```python
from build123d import *

# Parameters (mm, degrees)
SKETCH1_R                                       = 60.5
BOSS_EXTRUDE1_DEPTH                             = 5
SKETCH2_R                                       = 50
SKETCH2_R_2                                     = 45
BOSS_EXTRUDE2_DEPTH                             = 50
SKETCH3_W                                       = 9
SKETCH3_H                                       = 9
BOSS_EXTRUDE3_DEPTH                             = 1
SKETCH3_3_W                                     = 8
SKETCH3_3_H                                     = 9
BOSS_EXTRUDE4_DEPTH                             = 25
SKETCH4_W                                       = 25
SKETCH4_H                                       = 9
BOSS_EXTRUDE5_DEPTH                             = 5
BOSS_EXTRUDE7_DEPTH                             = 12.5
CSK_FOR_M3_FLAT_HEAD_MACHINE_SCREW1_D           = 3.4
CSK_FOR_M3_FLAT_HEAD_MACHINE_SCREW1_DEPTH       = 5
CSK_FOR_M3_FLAT_HEAD_MACHINE_SCREW1_CSINK_D     = 6.3
CSK_FOR_M3_FLAT_HEAD_MACHINE_SCREW1_CSINK_ANGLE = 90
CUT_EXTRUDE1_REACH                              = 132
SKETCH10_R                                      = 5


with BuildPart() as part:
    # Sketch1 → Boss-Extrude1 (new body)
    with BuildSketch(Plane(origin=(0, 0, 0), x_dir=(1, 0, 0), z_dir=(0, 1, 0))):
        Circle(SKETCH1_R)
        with BuildLine():
            Line((-14, -10.5), (14, -10.5))
            Line((14, -10.5), (35.078449216, -28.186918963))
            ThreePointArc((35.078449216, -28.186918963), (0, 45), (-35.078449216, -28.186918963))
            Line((-35.078449216, -28.186918963), (-14, -10.5))
        make_face(mode=Mode.SUBTRACT)
        with BuildLine():
            Line((-17.5, -23.5), (-23.628355545, -28.642300877))
            ThreePointArc((-23.628355545, -28.642300877), (0, -36.5), (23.628355545, -28.642300877))
            Line((23.628355545, -28.642300877), (17.5, -23.5))
            Line((17.5, -23.5), (-17.5, -23.5))
        make_face(mode=Mode.SUBTRACT)
    extrude(amount=BOSS_EXTRUDE1_DEPTH)

    # Sketch2 → Boss-Extrude2 (add)
    with BuildSketch(Plane(origin=(0, 5, 0), x_dir=(1, 0, 0), z_dir=(0, 1, 0))):
        Circle(SKETCH2_R)
        Circle(SKETCH2_R_2, mode=Mode.SUBTRACT)
    extrude(amount=BOSS_EXTRUDE2_DEPTH)

    # Sketch3 → Boss-Extrude3 (add)
    with BuildSketch(Plane(origin=(0, 5, 0), x_dir=(1, 0, 0), z_dir=(0, 1, 0))):
        with Locations((0, -15)):
            Rectangle(SKETCH3_W, SKETCH3_H)
    extrude(amount=BOSS_EXTRUDE3_DEPTH)

    # Sketch3<3> → Boss-Extrude4 (add)
    with BuildSketch(Plane(origin=(0, 5, 0), x_dir=(1, 0, 0), z_dir=(0, 1, 0))):
        with Locations((-8.5, -15)):
            Rectangle(SKETCH3_3_W, SKETCH3_3_H)
        with Locations((8.5, -15)):
            Rectangle(SKETCH3_3_W, SKETCH3_3_H)
    extrude(amount=BOSS_EXTRUDE4_DEPTH)

    # Sketch4 → Boss-Extrude5 (add)
    with BuildSketch(Plane(origin=(0, 30, 0), x_dir=(1, 0, 0), z_dir=(0, 1, 0))):
        with Locations((0, -15)):
            Rectangle(SKETCH4_W, SKETCH4_H)
    extrude(amount=BOSS_EXTRUDE5_DEPTH)

    # Sketch5 → Boss-Extrude7 (add, symmetric)
    with BuildSketch(Plane(origin=(0, 0, 0), x_dir=(0, 0, -1), z_dir=(1, 0, 0))):
        Polygon((41, 35), (32.5, 35), (32.5, 30), (46, 17), (46, 37), (41, 37), align=None)
    extrude(amount=BOSS_EXTRUDE7_DEPTH, both=True)

    # CSK for M3 Flat Head Machine Screw1
    with Locations(Plane(origin=(0, 5, 0), x_dir=(1, 0, 0), z_dir=(0, 1, 0))):
        with Locations((-36.842001616, 40.837077723), (36.842001616, 40.837077723), (36, -41.581245773), (-36.842001616, -40.837077723)):
            CounterSinkHole(CSK_FOR_M3_FLAT_HEAD_MACHINE_SCREW1_D / 2, CSK_FOR_M3_FLAT_HEAD_MACHINE_SCREW1_CSINK_D / 2, depth=CSK_FOR_M3_FLAT_HEAD_MACHINE_SCREW1_DEPTH, counter_sink_angle=CSK_FOR_M3_FLAT_HEAD_MACHINE_SCREW1_CSINK_ANGLE)

    # Sketch10 → Cut-Extrude1 (cut, up to next)
    with BuildSketch(Plane.XY.offset(69.5), mode=Mode.PRIVATE) as cut_extrude1_sk1:
        with Locations((0, 15)):
            Circle(SKETCH10_R)
    cut_extrude1_tool1 = extrude(cut_extrude1_sk1.sketch, amount=-CUT_EXTRUDE1_REACH, mode=Mode.PRIVATE) & part.part
    add(cut_extrude1_tool1.solids().sort_by_distance((0, 15, 69.5))[0], mode=Mode.SUBTRACT)


solid = part.part
```
For this review, take the finished solid that the model builds, in its own axes (mm). A direction names the side the tool comes from. Coordinates: 2 decimals unless noted, no trailing zeros. Write each loop counter-clockwise with the first axis right and the second up, starting at its lowest first coordinate (ties: lowest second). Pieces come first, ordered by that corner, then holes.
(1) Add section A-A on z = 0. Give the boundary of the cut face in (x, y).
(2) Add section D-D on x = -43. Give the boundary of the cut face in (y, z).
(3) Wall thickness on probe 1 along Z at (x, y) = (0.5, 47); probe 2 along Z at (x, y) = (0, 31); probe 3 along Z at (x, y) = (9, 3): over which ranges is each line inside the solid? List them lowest first.
(4) Add section B-B on y = 28. Give the boundary of the cut face in (x, z).
(5) Tool access review of faces 4 (the face through (0, 37, -43)), 5 (the face through (24.39, 2.46, 19.22)), 6 (the face through (0, 30, 15)): name each direction out of +Z, -Z, +X, -X, +Y, -Y from which nothing blocks a thin tool from reaching the whole face with its end or side.
(6) The part is to be moulded in two halves that separate along X. For faces 1 (the face through (-1.08, 10.12, 47.4)), 2 (the face through (-41, 55, -19)), 3 (the face through (47.69, 29.65, -15.02)), say which applies: +X half, -X half, draft (parallel to the pull), parting line (faces both ways), or undercut.
(7) Add section C-C on x = 0. Count the separate pieces of the cut face and the enclosed holes in it, then the cut area to 3 significant figures.
(8) For pin 1 Ø1 at (x, y) = (3.5, 14.5) entering from -Z; pin 2 Ø4 at (y, z) = (12.5, -46) entering from -X; pin 3 Ø12 at (y, z) = (28, -39.5) entering from +X; pin 4 Ø10 at (x, z) = (0.5, 16.5) entering from -Y, all flat-tipped, find the tip position at first contact; note any pin that passes through.
Answer sheet:
1. outline: (-60.5, 0) - (-45, 0) - (-45, 55) - (-50, 55) - (-50, 5) - (-60.5, 5) - close; (45, 0) - (60.5, 0) - (60.5, 5) - (50, 5) - (50, 55) - (45, 55) - close
2. outline: (0, -42.56) - (5, -42.56) - (5, -25.51) - (55, -25.51) - (55, -13.27) - (0, -13.27) - close; (0, 13.27) - (55, 13.27) - (55, 25.51) - (5, 25.51) - (5, 42.56) - (0, 42.56) - close
3. probe 1: z = -50 to -45, 45 to 50
3. probe 2: z = -50 to -32.5, 10.5 to 19.5, 45 to 50
3. probe 3: z = -59.83 to -44.09, 10.5 to 23.5, 35.46 to 59.83
4. outline: circle Ø100 at (0, 0); (-12.5, 10.5) - (-4.5, 10.5) - (-4.5, 19.5) - (-12.5, 19.5) - close; (4.5, 10.5) - (12.5, 10.5) - (12.5, 19.5) - (4.5, 19.5) - close; hole (-12.5, -43.23) - (-12.5, -34.58) - (12.5, -34.58) - (12.5, -43.23) arc R45 ccw (long way) to start
5. face 4: +Y
5. face 5: +Y, -Y
5. face 6: none
6. face 1: undercut
6. face 2: draft
6. face 3: parting line
7. separate pieces: 5
7. enclosed holes: 0
7. area: 912 mm2
8. pin 1: stops at z = -49.91
8. pin 2: stops at x = -23.75
8. pin 3: stops at x = 37.12
8. pin 4: stops at y = 0
